Geometry check sheet. Reference: the model listing, model coordinates, mm. Face numbers are marked on the shaded views. A direction names the side the tool comes from. Give positions to 0.01 mm unless a question says otherwise; leave off trailing zeros. Write each loop counter-clockwise with the first axis right and the second up, starting at its lowest first coordinate (ties: lowest second). Pieces come first, ordered by that corner, then holes.
(1) Thickness scan on line 1 along Z through (x, y) = (-18, -10.5); line 2 along X through (y, z) = (-16.25, -17.5); line 3 along X through (y, z) = (-1.25, -15). Record the ranges inside material, lowest first.
(2) Cross-section at A-A (z = -22). Record the boundary of the cut face in (x, y).
(3) Tool access check on the marked faces 1 and 2. Record the directions out of +Z, -Z, +X, -X, +Y, -Y that give a thin tool (end or side, any length) a straight path to the whole face; none if there is none.
(4) Cross-section at B-B (x = -60.5). Record the boundary of the cut face in (y, z), and give its area (3 significant figures).
(5) Depth check by flat-ended pin: P1, Ø5, axis at y = -7.5, z = -23.5, coming from the -X side; P2, Ø3, axis at y = -13, z = -5, coming from the +X side; P3, Ø12, axis at y = -18.5, z = -23, coming from the +X side. Enter the tip coordinate at first touch or a pass-through.
```python
from build123d import *

# Parameters (mm, degrees)
SKETCH13_R              = 1.651
BASE_FLANGE5_DEPTH      = 3.302
EDGE_FLANGE4_START      = -48.484504913
EDGE_FLANGE4_DEPTH      = 25.4
CUT_EXTRUDE4_DEPTH      = 4.699
CUT_EXTRUDE4_DEPTH_BACK = 36.068


# Read off the part's stored shape, not the designer's step: Edge-Flange4
# Sheet-metal steps are written as plain solids
with BuildPart() as part:
    # Sketch13 → Base-Flange5 (new body)
    with BuildSketch(Plane.XY):
        Polygon((-66.04, 0), (0, 0), (0, -23.797677877), (-74.918655736, -23.797677877), align=None)
        with Locations((-7.065339848, -12.296727665)):
            Circle(SKETCH13_R, mode=Mode.SUBTRACT)
    extrude(amount=-BASE_FLANGE5_DEPTH)

    # Edge-Flange4 outline → Edge-Flange4 (add)
    with BuildSketch(Plane(origin=(0, 0, 0), x_dir=(0.9369164518419233, -0.34955337542060905, 0), z_dir=(0.34955337542060905, 0.9369164518419232, 0)).offset(EDGE_FLANGE4_START)):
        with BuildLine():
            ThreePointArc((-65.17596248, 3.302), (-64.208829071, 0.967133409), (-61.87396248, 0))
            Line((-61.87396248, 0), (-61.87396248, 30.48))
            Line((-61.87396248, 30.48), (-65.17596248, 30.48))
            Line((-65.17596248, 30.48), (-65.17596248, 3.302))
        make_face()
    extrude(amount=EDGE_FLANGE4_DEPTH)

    # Sketch51 → Cut-Extrude4 (cut, two sides: drawn at the far end of the back side and taken through both)
    with BuildSketch(Plane.XY.offset(-CUT_EXTRUDE4_DEPTH_BACK)):
        Polygon((-66.04, 0), (-69.564327056, 0), (-69.133698124, 1.154225246), align=None)
    extrude(amount=CUT_EXTRUDE4_DEPTH + CUT_EXTRUDE4_DEPTH_BACK, mode=Mode.SUBTRACT)


solid = part.part
```
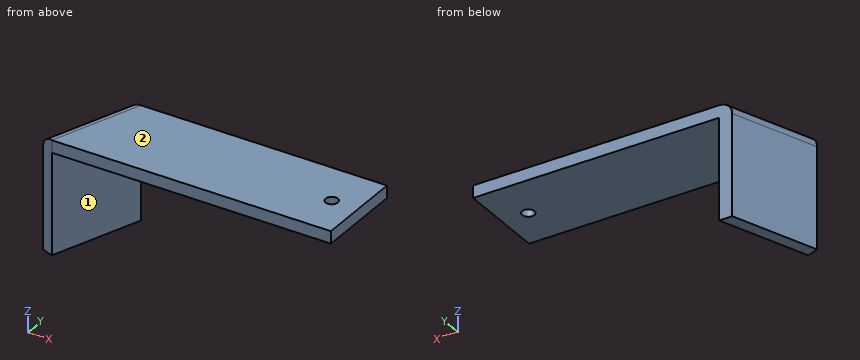
Reply:
1. line 1: z = -3.3 to 0
1. line 2: x = -75.63 to -72.1
1. line 3: x = -70.03 to -66.51
2. outline: (-78.01, -22.64) - (-74.92, -23.8) - (-66.04, 0) - (-69.56, 0) - close
3. face 1: -Z, +X, -Y
3. face 2: +Z, +X, -X, +Y, -Y
4. outline: (-23.8, -3.3) - (0, -3.3) - (0, 0) - (-23.8, 0) - close
4. area: 78.6 mm2
5. P1: stops at x = -73.3
5. P2: stops at x = -70.33
5. P3: stops at x = -70.7
